Can you work these out from the model? Positions are in its coordinate system, mm. A direction names the side the tool comes from. Round coordinates to 2 decimals unless told otherwise and drop trailing zeros. Loops run counter-clockwise (first coordinate to the right, second up) from the corner with the lowest first, then second, coordinate; pieces in that order, holes last. Notation, with made-up numbers: (26, -37) -> (57, -37) arc R21 ccw to (57, -31) -> close; hole circle Ø1 at (-19.75, -20). An arc over 180 degrees is marked (long way). Use a Markdown table: item, result.
from build123d import *

# Parameters (mm, degrees)
F0_W     = 215.9
F0_H     = 76.2
F1_DEPTH = 6.35
F2_W     = 6.35
F2_H     = 15.875
F2_H_2   = 9.525
F3_DEPTH = 6.35
F4_W     = 25.4
F4_H     = 6.35
F5_DEPTH = 6.351
F6_W     = 6.35
F6_H     = 9.525
F7_DEPTH = 6.35


with BuildPart() as f1:
    # F0 (on Front) → F1 (new body)
    with BuildSketch(Plane.XZ):
        with Locations((107.95, 38.1)):
            Rectangle(F0_W, F0_H)
    extrude(amount=F1_DEPTH)

    # F2 (on face) → F3 (cut, through all)
    with BuildSketch(Plane.XZ.offset(6.35)):
        with Locations((3.175, 58.7375)):
            Rectangle(F2_W, F2_H)
        with Locations((3.175, 33.3375)):
            Rectangle(F2_W, F2_H)
        with Locations((3.175, 11.1125)):
            Rectangle(F2_W, F2_H_2)
        with Locations((212.725, 11.1125)):
            Rectangle(F2_W, F2_H_2)
        with Locations((212.725, 33.3375)):
            Rectangle(F2_W, F2_H)
        with Locations((212.725, 58.7375)):
            Rectangle(F2_W, F2_H)
    extrude(amount=-F3_DEPTH, mode=Mode.SUBTRACT)

    # F4 (on face) → F5 (cut, through all)
    with BuildSketch(Plane.XZ.offset(6.35)):
        with Locations((12.7, 3.175)):
            Rectangle(F4_W, F4_H)
        with Locations((63.5, 3.175)):
            Rectangle(F4_W, F4_H)
        with Locations((114.3, 3.175)):
            Rectangle(F4_W, F4_H)
        with Locations((165.1, 3.175)):
            Rectangle(F4_W, F4_H)
        with Locations((215.9, 3.175)):
            Rectangle(F4_W, F4_H)
    extrude(amount=-F5_DEPTH, mode=Mode.SUBTRACT)

    # F6 (on face) → F7 (cut, through all)
    with BuildSketch(Plane.XZ.offset(6.35)):
        with Locations((212.725, 20.6375)):
            Rectangle(F6_W, F6_H)
        with Locations((212.725, 71.4375)):
            Rectangle(F6_W, F6_H)
    extrude(amount=-F7_DEPTH, mode=Mode.SUBTRACT)


solid = f1.part
1. I want a section at C-C (z = 60.5). Please give me the cut outline in (x, y).
Answer sheet:
| item | result |
|---|---|
| outline | (6.35, -6.35) -> (209.55, -6.35) -> (209.55, 0) -> (6.35, 0) -> close |
2. Will these pins go through, and if not, where does the flat tip stop? pin 1 Ø3 at (y, z) = (-4, 64.5) entering from -X; pin 2 Ø3 at (x, y) = (18.5, -2) entering from -Z; pin 3 Ø1.5 at (x, y) = (97, -4.5) entering from -Z; pin 4 Ø3 at (y, z) = (-2, 4.5) entering from +X.
Answer sheet:
| item | result |
|---|---|
| pin 1 | stops at x = 6.35 |
| pin 2 | stops at z = 6.35 |
| pin 3 | stops at z = 0 |
| pin 4 | stops at x = 203.2 |
3. I need wall thicknesses on line 1 (X direction, y = -3, z = 56); line 2 (Z direction, x = 207.5, y = -3.75); line 3 (X direction, y = -5.5, z = 25). Which ranges of each line are inside material? Lowest first, please.
Answer sheet:
| item | result |
|---|---|
| line 1 | x = 6.35 to 209.55 |
| line 2 | z = 6.35 to 76.2 |
| line 3 | x = 0 to 209.55 |
4. Which directions (+Z, -Z, +X, -X, +Y, -Y) give clear straight access to the entire face, cutting with the end or side of a thin tool? Please do faces 1 (the flat face through (3, -3, 15.875)), 2 (the flat face through (209.55, -3, 63)), 3 (the flat face through (209.55, -3, 24)), 4 (the flat face through (165, -3, 6.35)).
Answer sheet:
| item | result |
|---|---|
| face 1 | -Z, -X, +Y, -Y |
| face 2 | +Z, +X, +Y, -Y |
| face 3 | -Z, +X, +Y, -Y |
| face 4 | -Z, +Y, -Y |
5. I want a section at B-B (x = 123.5). Please give me the cut outline in (y, z), plus the area to 3 significant figures.
Answer sheet:
| item | result |
|---|---|
| outline | (-6.35, 6.35) -> (0, 6.35) -> (0, 76.2) -> (-6.35, 76.2) -> close |
| area | 444 mm² |
6. If we mould it in two halves opening along X, with no side actions, what happens to faces 5 (the flat face through (76.2, -3, 3)), 6 (the flat face through (25.4, -3, 3)), 7 (the flat face through (215.9, -3, 46))? For each: +X half, -X half, draft (parallel to the pull), parting line (faces both ways), or undercut.
Answer sheet:
| item | result |
|---|---|
| face 5 | undercut |
| face 6 | -X half |
| face 7 | +X half |
